```python
from build123d import *

# Parameters (mm, degrees)
ESBO_O2_W                = 53
ESBO_O2_H                = 100
RESSALTO_EXTRUS_O1_DEPTH = 3
ESBO_O3_R                = 2
CORTE_EXTRUS_O1_DEPTH    = 10
ESBO_O4_R                = 2.5
CORTE_EXTRUS_O3_DEPTH    = 10
ESBO_O5_R                = 2
CORTE_EXTRUS_O4_DEPTH    = 10
ESBO_O6_W                = 3
ESBO_O6_H                = 30
CORTE_EXTRUS_O8_DEPTH    = 10


with BuildPart() as part:
    # Esboço2 → Ressalto-extrusão1 (new body)
    with BuildSketch(Plane(origin=(0, 0, 0), x_dir=(1, 0, 0), z_dir=(0, 1, 0))):
        with Locations((-26.520406012, 50)):
            Rectangle(ESBO_O2_W, ESBO_O2_H)
    extrude(amount=RESSALTO_EXTRUS_O1_DEPTH)

    # Esboço3 → Corte-extrusão1 (cut)
    with BuildSketch(Plane(origin=(0, 3, 0), x_dir=(1, 0, 0), z_dir=(0, 1, 0))):
        with Locations(Location((-25, 10, 0), (0, 0, 270))):
            Circle(ESBO_O3_R)
    extrude(amount=-CORTE_EXTRUS_O1_DEPTH, mode=Mode.SUBTRACT)

    # Esboço4 → Corte-extrusão3 (cut)
    with BuildSketch(Plane(origin=(0, 3, 0), x_dir=(1, 0, 0), z_dir=(0, 1, 0))):
        with Locations(Location((-37, 73.5, 0), (0, 0, 270))):
            Circle(ESBO_O4_R)
    extrude(amount=-CORTE_EXTRUS_O3_DEPTH, mode=Mode.SUBTRACT)

    # Esboço5 → Corte-extrusão4 (cut)
    with BuildSketch(Plane(origin=(0, 3, 0), x_dir=(1, 0, 0), z_dir=(0, 1, 0))):
        with Locations(Location((-26.520406012, 90, 0), (0, 0, 270))):
            Circle(ESBO_O5_R)
    extrude(amount=-CORTE_EXTRUS_O4_DEPTH, mode=Mode.SUBTRACT)

    # Esboço6 → Corte-extrusão8 (cut)
    with BuildSketch(Plane(origin=(0, 3, 0), x_dir=(1, 0, 0), z_dir=(0, 1, 0))):
        with Locations((-44.419461936, 35)):
            Rectangle(ESBO_O6_W, ESBO_O6_H)
        with Locations((-38.419461936, 35)):
            Rectangle(ESBO_O6_W, ESBO_O6_H)
        with Locations((-32.419461936, 35)):
            Rectangle(ESBO_O6_W, ESBO_O6_H)
        with Locations((-26.419461936, 35)):
            Rectangle(ESBO_O6_W, ESBO_O6_H)
    extrude(amount=-CORTE_EXTRUS_O8_DEPTH, mode=Mode.SUBTRACT)


solid = part.part
```
Source: CAD feature listing. Evaluate the final solid. Frame: model axes, mm. Round coordinates to 2 decimals unless told otherwise and drop trailing zeros. Order: outer loops, then holes, each group sorted by start corner. A loop starts at its lowest first (then second) coordinate and runs counter-clockwise, first axis right, second up. Notation, with made-up numbers: (-22, -36.75) -> (31, -36.75) arc R34 cw to (31, -2.75) -> close; hole circle Ø2 at (-3, -32.75). An arc over 180 degrees is marked (long way). Use CSV: the item, a comma, the result in double quotes.
(1) Section B-B on z = -43. Return the cut outline in (x, y).
Report:
outline,"(-53.02, 0) -> (-45.92, 0) -> (-45.92, 3) -> (-53.02, 3) -> close; (-42.92, 0) -> (-39.92, 0) -> (-39.92, 3) -> (-42.92, 3) -> close; (-36.92, 0) -> (-33.92, 0) -> (-33.92, 3) -> (-36.92, 3) -> close; (-30.92, 0) -> (-27.92, 0) -> (-27.92, 3) -> (-30.92, 3) -> close; (-24.92, 0) -> (-0.02, 0) -> (-0.02, 3) -> (-24.92, 3) -> close"
(2) Section C-C on z = -10. Return the cut outline in (x, y), and give its area (3 significant figures).
Report:
outline,"(-53.02, 0) -> (-27, 0) -> (-27, 3) -> (-53.02, 3) -> close; (-23, 0) -> (-0.02, 0) -> (-0.02, 3) -> (-23, 3) -> close"
area,"147 mm^2"
(3) Section A-A on x = -32. Return the cut outline in (y, z).
Report:
outline,"(0, -100) -> (3, -100) -> (3, -50) -> (0, -50) -> close; (0, -20) -> (3, -20) -> (3, 0) -> (0, 0) -> close"
(4) Ray query, L1, parallel to X at y = 2.15, z = -47; L2, parallel to X at y = 2.2, z = -73.5; L3, parallel to X at y = 2.15, z = -90. Return the intervals inside material, ascending.
Report:
L1,"-53.02 to -45.92, -42.92 to -39.92, -36.92 to -33.92, -30.92 to -27.92, -24.92 to -0.02"
L2,"-53.02 to -39.5, -34.5 to -0.02"
L3,"-53.02 to -28.52, -24.52 to -0.02"
(5) Section D-D on x = -38. Return the cut outline in (y, z).
Report:
outline,"(0, -100) -> (3, -100) -> (3, -75.79) -> (0, -75.79) -> close; (0, -71.21) -> (3, -71.21) -> (3, -50) -> (0, -50) -> close; (0, -20) -> (3, -20) -> (3, 0) -> (0, 0) -> close"
(6) Pull-direction query (Z, two-part tool) for faces 1 (the face through (-27, 1, -100)), 2 (the face through (-38, 2, -20)), 3 (the face through (-27, 1, 0)); classes: +Z half, -Z half, draft (parallel to the pull), parting line (faces both ways), or undercut.
Report:
face 1,"-Z half"
face 2,"undercut"
face 3,"+Z half"
(7) First-contact query: pin 1 Ø4 at (x, z) = (-37, -73.5) entering from +Y. Flat tip, straight axial feed; report the tip coordinate or a pass-through.
Report:
pin 1,"through"
